Input: part model. Units: mm. Frame: model coordinates. A direction names the side the tool comes from. Give positions to 0.01 mm unless a question says otherwise; leave off trailing zeros. Loops run counter-clockwise (first coordinate to the right, second up) from the corner with the lowest first, then second, coordinate; pieces in that order, holes last. Notation, with made-up numbers: M 18.25,62 L 33.25,62 A24 ccw 33.25,93 Z; hole C 63,-1.5 d2. An arc over 180 degrees is marked long. Answer as a JSON object with one key per item and string values. Group by question number.
1) Section query B-B on z = -56.9. Return loops of the section in (x, y), plus the area to 3 significant figures.
2) Section query C-C on y = 2.4. Return loops of the section in (x, z), plus the area to 3 significant figures.
3) Draft query along Z for faces 1 (the cylindrical face through (36.982, 1.479, -57.173)), 2 (the flat face through (25, 1, -65)), 3 (the flat face through (20, 1, -3)). Return one class per face: +Z half, -Z half, draft (parallel to the pull), parting line (faces both ways), or undercut.
4) Section query D-D on x = 20. Return loops of the section in (y, z), plus the area to 3 significant figures.
5) Section query A-A on x = 34.9. Return loops of the section in (y, z), plus the area to 3 significant figures.
6) Access query for faces 4 (the cylindrical face through (26, 1.48, -24.43)), 5 (the flat face through (15, 1, -1)), 6 (the flat face through (20, 1, -63)), 7 (the flat face through (0, 1, -33)). Directions: +Z, -Z, +X, -X, +Y, -Y. A direction counts if a zero-diameter tool reaches every point of the face in a straight line with its end or side. Return the directions, or none.
7) Ray query, L1, parallel to X at y = 1, z = -56.9; L2, parallel to X at y = 1.1, z = -9.1; L3, parallel to X at y = 0.35, z = -55.5. Return the intervals inside material, ascending.
8) First-contact query: P1, Ø1.5, axis at x = 21, y = 2, coming from the +Z side; P2, Ø4, axis at x = 20, z = -9.1, coming from the -Y side; P3, Ø0.9, axis at x = 18, y = 1, coming from the -Z side. Flat tips, straight axial feed; report the tip coordinate or a pass-through.
from build123d import *

# Parameters (mm, degrees)
SKETCH1_R           = 2.1
BOSS_EXTRUDE1_DEPTH = 3
SKETCH3_W           = 15
SKETCH3_H           = 20
CUT_EXTRUDE1_DEPTH  = 78.233412459
FILLET1_R           = 5


with BuildPart() as part:
    # Sketch1 → Boss-Extrude1 (new body)
    with BuildSketch(Plane(origin=(0, 0, 0), x_dir=(1, 0, 0), z_dir=(0, 1, 0))):
        Polygon((0, 0), (15, 0), (15, 3), (25, 3), (25, 0), (40, 0), (40, 66), (25, 66), (25, 63), (15, 63), (15, 66), (0, 66), align=None)
        with Locations(Location((34.9, 56.9, 0), (0, 0, 270))):
            Circle(SKETCH1_R, mode=Mode.SUBTRACT)
        with Locations(Location((20, 9.1, 0), (0, 0, 270))):
            Circle(SKETCH1_R, mode=Mode.SUBTRACT)
        with Locations(Location((5.1, 56.9, 0), (0, 0, 270))):
            Circle(SKETCH1_R, mode=Mode.SUBTRACT)
    extrude(amount=BOSS_EXTRUDE1_DEPTH)

    # Sketch3 → Cut-Extrude1 (cut, through all)
    with BuildSketch(Plane(origin=(0, 3, 0), x_dir=(1, 0, 0), z_dir=(0, 1, 0))):
        with Locations((20, 33)):
            Rectangle(SKETCH3_W, SKETCH3_H)
    extrude(amount=-CUT_EXTRUDE1_DEPTH, mode=Mode.SUBTRACT)

    # Fillet1
    fillet1_edges = [part.edges().sort_by_distance(p)[0] for p in [
        (12.5, 1.5, -23),
        (12.5, 1.5, -43),
        (27.5, 1.5, -43),
        (27.5, 1.5, -23),
    ]]
    fillet(fillet1_edges, radius=FILLET1_R)


solid = part.part
Output:
{
 "1": {"outline": "M 0,0 L 3,0 L 3,3 L 0,3 Z; M 7.2,0 L 32.8,0 L 32.8,3 L 7.2,3 Z; M 37,0 L 40,0 L 40,3 L 37,3 Z", "area": "94.8 mm^2"},
 "2": {"outline": "M 0,-66 L 15,-66 L 15,-63 L 25,-63 L 25,-66 L 40,-66 L 40,0 L 25,0 L 25,-3 L 15,-3 L 15,0 L 0,0 Z; hole C 5.1,-56.9 d4.2; hole M 12.5,-38 A5 ccw 17.5,-43 L 22.5,-43 A5 ccw 27.5,-38 L 27.5,-28 A5 ccw 22.5,-23 L 17.5,-23 A5 ccw 12.5,-28 Z; hole C 20,-9.1 d4.2; hole C 34.9,-56.9 d4.2", "area": "2,260 mm^2"},
 "3": {"face 1": "undercut", "face 2": "draft", "face 3": "+Z half"},
 "4": {"outline": "M 0,-63 L 3,-63 L 3,-43 L 0,-43 Z; M 0,-23 L 3,-23 L 3,-11.2 L 0,-11.2 Z; M 0,-7 L 3,-7 L 3,-3 L 0,-3 Z", "area": "107 mm^2"},
 "5": {"outline": "M 0,-66 L 3,-66 L 3,-59 L 0,-59 Z; M 0,-54.8 L 3,-54.8 L 3,0 L 0,0 Z", "area": "185 mm^2"},
 "6": {"face 4": "+Y, -Y", "face 5": "+Z, +Y, -Y", "face 6": "-Z, +Y, -Y", "face 7": "+Z, -Z, -X, +Y, -Y"},
 "7": {"L1": "x = 0 to 3, 7.2 to 32.8, 37 to 40", "L2": "x = 0 to 17.9, 22.1 to 40", "L3": "x = 0 to 3.53, 6.67 to 33.33, 36.47 to 40"},
 "8": {"P1": "stops at z = -3", "P2": "passes through", "P3": "stops at z = -63"}
}
